Geometry check sheet. Reference: the model listing, model coordinates, mm. A direction names the side the tool comes from. Round coordinates to 2 decimals unless told otherwise and drop trailing zeros. Order: outer loops, then holes, each group sorted by start corner. A loop starts at its lowest first (then second) coordinate and runs counter-clockwise, first axis right, second up. Notation, with made-up numbers: (75, -3.5) - (89, -3.5) arc R9 ccw to (89, 7.5) - close; hole circle Ø4 at (-37.75, 17). An arc over 180 degrees is marked (long way). Answer as CSV lines item,"result". Start each with the question number.
Solid Edge part; units mm, degrees
sketch "Sketch1" plane through (0, 0, 0) normal (0, -1, 0) x (1, 0, 0)
  line L0 (10.9652, -11.6239) -> (-49.0348, -11.6239)
  line L1 (-49.0348, -11.6239) -> (-49.0348, -31.6239)
  line L2 (-49.0348, -31.6239) -> (10.9652, -31.6239)
  line L3 (10.9652, -31.6239) -> (10.9652, -11.6239)
extrude "Protrusion1" add sketch "Sketch1" against normal blind 60
sketch "Sketch2" plane through (-19.0348, 30, -11.6239) normal (0, 0, 1) x (1, 0, 0)
  line L0 (-20, -20) -> (20, -20)
  line L1 (20, -20) -> (20, 20)
  line L2 (20, 20) -> (-20, 20)
  line L3 (-20, 20) -> (-20, -20)
extrude "ExtrudedProtrusion_2" add sketch "Sketch2" along normal blind 50
sketch "Sketch3" plane through (-19.0348, 10, 13.3761) normal (0, -1, 0) x (1, 0, 0)
  line L0 (0, 25) -> (-20, -25)
  line L1 (-20, -25) -> (-20, 25)
  line L2 (-20, 25) -> (0, 25)
  line L3 (20, 25) -> (0, 25)
  line L4 (0, 25) -> (20, -25)
  line L5 (20, -25) -> (20, 25)
extrude "ExtrudedCutout_1" cut sketch "Sketch3" against normal blind 103.1734
sketch "Sketch4" plane through (10.9652, 30, -21.6239) normal (1, 0, 0) x (0, 1, 0)
  line L0 (0, 60) -> (-20, 10)
  line L1 (-20, 10) -> (-20, 60)
  line L2 (-20, 60) -> (0, 60)
  line L3 (0, 60) -> (20, 10)
  line L4 (20, 10) -> (20, 60)
  line L5 (20, 60) -> (0, 60)
extrude "ExtrudedCutout_2" cut sketch "Sketch4" against normal blind 271.3567
1. Thickness scan on probe 1 along Z at (x, y) = (-40.5, 55); probe 2 along Y at (x, z) = (-24, -9.5); probe 3 along Y at (x, z) = (-21, 33). Record the ranges inside material, lowest first.
2. Access from +Z, -Z, +X, -X, +Y, -Y to the whole of each face (thin tool, end or side, straight path). Record for faces 1 (the face through (-18.6, 9.6, -11.624)), 2 (the face through (-18.755, 17.918, 8.171)).
3. Section check B-B on y = 27. Record the boundary of the cut face in (x, z).
4. Go/stop test with flat-tipped pins: pin 1 Ø4 at (x, z) = (-21.5, -2) entering from +Y; pin 2 Ø6 at (x, z) = (-18, -8) entering from +Y. Record where each tip stops, or that it passes through.
5. Section check A-A on x = -33. Record the boundary of the cut face in (y, z), plus the area to 3 significant figures.
6. Section check C-C on z = 2.5. Record the boundary of the cut face in (x, y).
7. Section check D-D on y = 5.5. Record the boundary of the cut face in (x, z).
Numbers:
1,probe 1,"z = -31.62 to -11.62"
1,probe 2,"y = 10.85 to 49.15"
1,probe 3,"y = 27.85 to 32.15"
2,face 1,"+Z"
2,face 2,"+Z, +X, -X, -Y"
3,outline,"(-49.03, -31.62) - (10.97, -31.62) - (10.97, -11.62) - (0.97, -11.62) - (-16.03, 30.88) - (-22.03, 30.88) - (-39.03, -11.62) - (-49.03, -11.62) - close"
4,pin 1,"stops at y = 46.95"
4,pin 2,"stops at y = 49.75"
5,outline,"(0, -31.62) - (60, -31.62) - (60, -11.62) - (50, -11.62) - (43.97, 3.46) - (16.03, 3.46) - (10, -11.62) - (0, -11.62) - close"
5,area,"1,710 mm2"
6,outline,"(-33.39, 15.65) - (-4.68, 15.65) - (-4.68, 44.35) - (-33.39, 44.35) - close"
7,outline,"(-49.03, -31.62) - (10.97, -31.62) - (10.97, -11.62) - (-49.03, -11.62) - close"
